```python
from build123d import *

# Parameters (mm, degrees)
ESQUISSE1_W             = 1182
ESQUISSE1_H             = 60
BOSS_EXTRU_1_DEPTH      = 24
BOSS_EXTRU_2_DEPTH      = 30
BOSS_EXTRU_3_START      = -1212
BOSS_EXTRU_3_DEPTH      = 30
CHANFREIN1_SIZE         = 5
ENL_V_MAT_EXTRU_1_DEPTH = 15


with BuildPart() as part:
    # Esquisse1 → Boss.-Extru.1 (new body)
    with BuildSketch(Plane.XY):
        with Locations((591, 30)):
            Rectangle(ESQUISSE1_W, ESQUISSE1_H)
    extrude(amount=BOSS_EXTRU_1_DEPTH)

    # Esquisse2 → Boss.-Extru.2 (add)
    with BuildSketch(Plane.ZY):
        with BuildLine():
            Line((4, 15), (4, 45))
            ThreePointArc((4, 45), (12, 53), (20, 45))
            Line((20, 45), (20, 15))
            ThreePointArc((20, 15), (12, 7), (4, 15))
        make_face()
    extrude(amount=BOSS_EXTRU_2_DEPTH)

    # Esquisse2<2> → Boss.-Extru.3 (add)
    with BuildSketch(Plane.ZY.offset(BOSS_EXTRU_3_START)):
        with BuildLine():
            Line((4, 15), (4, 45))
            ThreePointArc((4, 45), (12, 53), (20, 45))
            Line((20, 45), (20, 15))
            ThreePointArc((20, 15), (12, 7), (4, 15))
        make_face()
    extrude(amount=BOSS_EXTRU_3_DEPTH)

    # Chanfrein1
    chanfrein1_edges = [part.edges().sort_by_distance(p)[0] for p in [
        (591, 60, 24),
        (591, 60, 0),
        (591, 0, 0),
        (591, 0, 24),
    ]]
    chamfer(chanfrein1_edges, length=CHANFREIN1_SIZE)

    # Esquisse3 → Enlèv. mat.-Extru.1 (cut)
    with BuildSketch(Plane(origin=(0, 60, 0), x_dir=(1, 0, 0), z_dir=(0, 1, 0))):
        with BuildLine():
            Line((483, -7), (495, -7))
            ThreePointArc((495, -7), (500, -12), (495, -17))
            Line((495, -17), (483, -17))
            ThreePointArc((483, -17), (478, -12), (483, -7))
        make_face()
        with BuildLine():
            Line((381, -7), (393, -7))
            ThreePointArc((393, -7), (398, -12), (393, -17))
            Line((393, -17), (381, -17))
            ThreePointArc((381, -17), (376, -12), (381, -7))
        make_face()
        with BuildLine():
            Line((279, -7), (291, -7))
            ThreePointArc((291, -7), (296, -12), (291, -17))
            Line((291, -17), (279, -17))
            ThreePointArc((279, -17), (274, -12), (279, -7))
        make_face()
        with BuildLine():
            Line((177, -7), (189, -7))
            ThreePointArc((189, -7), (194, -12), (189, -17))
            Line((189, -17), (177, -17))
            ThreePointArc((177, -17), (172, -12), (177, -7))
        make_face()
        with BuildLine():
            Line((75, -7), (87, -7))
            ThreePointArc((87, -7), (92, -12), (87, -17))
            Line((87, -17), (75, -17))
            ThreePointArc((75, -17), (70, -12), (75, -7))
        make_face()
        with BuildLine():
            Line((585, -7), (597, -7))
            ThreePointArc((597, -7), (602, -12), (597, -17))
            Line((597, -17), (585, -17))
            ThreePointArc((585, -17), (580, -12), (585, -7))
        make_face()
        with BuildLine():
            Line((1107, -7), (1095, -7))
            ThreePointArc((1095, -7), (1090, -12), (1095, -17))
            Line((1095, -17), (1107, -17))
            ThreePointArc((1107, -17), (1112, -12), (1107, -7))
        make_face()
        with BuildLine():
            Line((1005, -7), (993, -7))
            ThreePointArc((993, -7), (988, -12), (993, -17))
            Line((993, -17), (1005, -17))
            ThreePointArc((1005, -17), (1010, -12), (1005, -7))
        make_face()
        with BuildLine():
            Line((903, -7), (891, -7))
            ThreePointArc((891, -7), (886, -12), (891, -17))
            Line((891, -17), (903, -17))
            ThreePointArc((903, -17), (908, -12), (903, -7))
        make_face()
        with BuildLine():
            Line((801, -7), (789, -7))
            ThreePointArc((789, -7), (784, -12), (789, -17))
            Line((789, -17), (801, -17))
            ThreePointArc((801, -17), (806, -12), (801, -7))
        make_face()
        with BuildLine():
            Line((699, -7), (687, -7))
            ThreePointArc((687, -7), (682, -12), (687, -17))
            Line((687, -17), (699, -17))
            ThreePointArc((699, -17), (704, -12), (699, -7))
        make_face()
    extrude(amount=-ENL_V_MAT_EXTRU_1_DEPTH, mode=Mode.SUBTRACT)


solid = part.part
```
CAD build for the part. Positions are in the model's coordinates, mm. A direction names the side the tool comes from. Round coordinates to 2 decimals unless told otherwise and drop trailing zeros. Order: outer loops, then holes, each group sorted by start corner. A loop starts at its lowest first (then second) coordinate and runs counter-clockwise, first axis right, second up.
Item 1: Tool access for faces 1 (the face through (-15, 30, 4)), 2 (the face through (1197, 30, 4)), 3 (the face through (-15, 30, 20)), 4 (the face through (0, 29.6, 3.8)), 5 (the face through (1182, 29.6, 3.8)): list every direction of +Z, -Z, +X, -X, +Y, -Y with a clear straight run to the whole face (end or side of a thin tool).
Item 2: Saw through at B-B on y = 28.5. Write the cut outline in (x, z).
Item 3: Saw through at A-A on x = 972. Write the cut outline in (y, z), then the cut area to 3 significant figures.
Item 4: Probe line 1 along X through (y, z) = (11, 4.5); line 2 along Y through (x, z) = (861.5, 19.75); line 3 along Y through (x, z) = (1137, 19.5). List the from-to ranges inside material, lowest first.
Item 5: Pin check, flat tip, straight feed: pin 1 (5 mm diameter, centred on x = 488.5, z = 10.5, fed in from +Y). Stop position of the tip, or through.
Reported:
1. face 1: -Z, -X, +Y, -Y
1. face 2: -Z, +X, +Y, -Y
1. face 3: +Z, -X, +Y, -Y
1. face 4: -X
1. face 5: +X
2. outline: (-30, 4) - (0, 4) - (0, 0) - (1182, 0) - (1182, 4) - (1212, 4) - (1212, 20) - (1182, 20) - (1182, 24) - (0, 24) - (0, 20) - (-30, 20) - close
3. outline: (0, 5) - (5, 0) - (55, 0) - (60, 5) - (60, 19) - (55, 24) - (5, 24) - (0, 19) - close
3. area: 1,390 mm2
4. line 1: x = 0 to 1182
4. line 2: y = 0.75 to 59.25
4. line 3: y = 0.5 to 59.5
5. pin 1: stops at y = 45
